from build123d import *

# Parameters (mm, degrees)
F0_W     = 50
F0_H     = 50
F1_DEPTH = 50
F2_R     = 5.916819
F2_R_2   = 6.667028
F3_DEPTH = 50.001
F4_W     = 14.457899
F4_H     = 11.871012
F5_DEPTH = 25


with BuildPart() as f1:
    # F0 (on Top) → F1 (new body)
    with BuildSketch(Plane.XY):
        with Locations((-5.997218, 2.292054)):
            Rectangle(F0_W, F0_H)
    extrude(amount=F1_DEPTH)

    # F2 (on face) → F3 (cut, through all)
    with BuildSketch(Plane.XZ.offset(22.707946)):
        with Locations((-21.676753, 40.365946)):
            Circle(F2_R)
        with Locations((8.427949, 9.634061)):
            Circle(F2_R_2)
    extrude(amount=-F3_DEPTH, mode=Mode.SUBTRACT)

    # F4 (on face) → F5 (join)
    with BuildSketch(Plane.XY.offset(50)):
        with Locations((-7.228949, 5.935506)):
            Rectangle(F4_W, F4_H)
    extrude(amount=F5_DEPTH)


solid = f1.part
The model under review builds one solid part; all positions refer to its coordinate system, in mm. A direction names the side the tool comes from. Give positions to 0.01 mm unless a question says otherwise; leave off trailing zeros. Order: outer loops, then holes, each group sorted by start corner. A loop starts at its lowest first (then second) coordinate and runs counter-clockwise, first axis right, second up. Notation, with made-up numbers: (0, -16.75) -> (47, -16.75) arc R13 ccw to (47, 6.25) -> close; hole circle Ø11 at (-1.75, 64). An arc over 180 degrees is marked (long way). Write item = value, one per line. Start each with the question number.
(1) Take a section at C-C (y = -17). Write out the cut boundary in (x, z).
(2) For pin 1 Ø3.5 at (y, z) = (4.5, 62.5) entering from -X; pin 2 Ø7 at (x, z) = (-5.5, 58) entering from -Y; pin 3 Ø3.5 at (y, z) = (4, 63.5) entering from +X, all flat-tipped, find the tip position at first contact; note any pin that passes through.
(3) Tool access review of faces 1 (the flat face through (-7, 0, 62)), 2 (the flat face through (0, 6, 62)), 3 (the flat face through (-7, 11.871, 62)), 4 (the flat face through (-14.458, 6, 62)): name each direction out of +Z, -Z, +X, -X, +Y, -Y from which nothing blocks a thin tool from reaching the whole face with its end or side.
(4) Draft analysis for pull direction X (two halves, no side actions). For faces 5 (the cylindrical face through (7.56, 1.942, 16.244)), 6 (the cylindrical face through (-18, 2, 45)), 7 (the flat face through (-30.997, 2, 25)), 8 (the flat face through (-6, -3, 50)), state which applies: +X half, -X half, draft (parallel to the pull), parting line (faces both ways), or undercut.
(5) Take a section at D-D (z = 52.5). Write out the cut boundary in (x, y).
(6) For L1, parallel to Z at x = -7, y = -19; L2, parallel to Z at x = -24.5, y = 3; L3, parallel to X at y = 10, z = 42, list the stretches that pass through material, from the lowest coordinate up. Write a range as from..to.
(7) Take a section at B-B (x = 6.5). Write out the cut boundary in (y, z), plus the area to 3 significant figures.
(8) Take a section at A-A (x = -2). Write out the cut boundary in (y, z), plus the area to 3 significant figures.
Returned:
q1.outline = (-31, 0) -> (19, 0) -> (19, 50) -> (-31, 50) -> close; hole circle Ø11.83 at (-21.68, 40.37); hole circle Ø13.33 at (8.43, 9.63)
q2.pin_1 = -14.46
q2.pin_2 = 0
q2.pin_3 = 0
q3.face_1 = +Z, +X, -X, -Y
q3.face_2 = +Z, +X, +Y, -Y
q3.face_3 = +Z, +X, -X, +Y
q3.face_4 = +Z, -X, +Y, -Y
q4.face_5 = undercut
q4.face_6 = undercut
q4.face_7 = -X half
q4.face_8 = draft
q5.outline = (-14.46, 0) -> (0, 0) -> (0, 11.87) -> (-14.46, 11.87) -> close
q6.L1 = 0..50
q6.L2 = 0..35.17, 45.57..50
q6.L3 = -31..-27.36, -15.99..19
q7.outline = (-22.71, 0) -> (27.29, 0) -> (27.29, 3.25) -> (-22.71, 3.25) -> close; (-22.71, 16.02) -> (27.29, 16.02) -> (27.29, 50) -> (-22.71, 50) -> close
q7.area = 1,860 mm²
q8.outline = (-22.71, 0) -> (27.29, 0) -> (27.29, 50) -> (11.87, 50) -> (11.87, 75) -> (0, 75) -> (0, 50) -> (-22.71, 50) -> close
q8.area = 2,800 mm²
